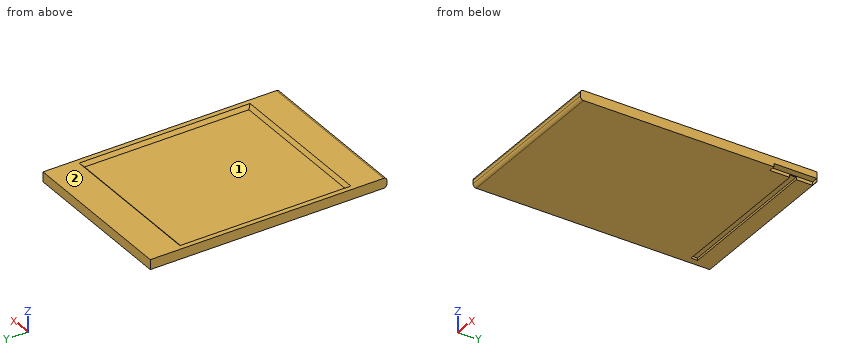
```python
from build123d import *

# Parameters (mm, degrees)
CROQUIS1_W              = 500
CROQUIS1_H              = 720
SALIENTE_EXTRUIR1_DEPTH = 30
CROQUIS2_W              = 450
CROQUIS2_H              = 500
CORTAR_EXTRUIR1_DEPTH   = 10
CHAFL_N1_SIZE           = 10
CHAFL_N2_SIZE           = 10
REDONDEO2_R             = 10
REDONDEO3_R             = 10
CROQUIS11_W             = 480
CROQUIS11_H             = 20
CORTAR_EXTRUIR5_DEPTH   = 7
CROQUIS12_W             = 10
CROQUIS12_H             = 130
CORTAR_EXTRUIR6_DEPTH   = 20


with BuildPart() as part:
    # Croquis1 → Saliente-Extruir1 (new body)
    with BuildSketch(Plane.XY):
        Rectangle(CROQUIS1_W, CROQUIS1_H)
    extrude(amount=SALIENTE_EXTRUIR1_DEPTH)

    # Croquis2 → Cortar-Extruir1 (cut)
    with BuildSketch(Plane.XY.offset(30)):
        Rectangle(CROQUIS2_W, CROQUIS2_H)
    extrude(amount=-CORTAR_EXTRUIR1_DEPTH, mode=Mode.SUBTRACT)

    # Chaflán1
    chafl_n1_edges = [part.edges().sort_by_distance(p)[0] for p in [
        (0, 250, 30),
    ]]
    chamfer(chafl_n1_edges, length=CHAFL_N1_SIZE - 0.0001)  # a hair under: the kernel refuses the full size

    # Chaflán2
    chafl_n2_edges = [part.edges().sort_by_distance(p)[0] for p in [
        (225, 4.99995, 30),
        (0, -250, 30),
        (-225, 4.99995, 30),
    ]]
    chamfer(chafl_n2_edges, length=CHAFL_N2_SIZE - 0.0001)  # a hair under: the kernel refuses the full size

    # Redondeo2
    redondeo2_edges = [part.edges().sort_by_distance(p)[0] for p in [
        (0, -360, 30),
    ]]
    fillet(redondeo2_edges, radius=REDONDEO2_R)

    # Redondeo3
    redondeo3_edges = [part.edges().sort_by_distance(p)[0] for p in [
        (0, -360, 0),
    ]]
    fillet(redondeo3_edges, radius=REDONDEO3_R)

    # Croquis11 → Cortar-Extruir5 (cut)
    with BuildSketch(Plane(origin=(0, 0, 0), x_dir=(-1, 0, 0), z_dir=(0, 0, -1))):
        with Locations((-10, 300)):
            Rectangle(CROQUIS11_W, CROQUIS11_H)
    extrude(amount=-CORTAR_EXTRUIR5_DEPTH, mode=Mode.SUBTRACT)

    # Croquis12 → Cortar-Extruir6 (cut)
    with BuildSketch(Plane(origin=(250, 0, 0), x_dir=(0, 0, -1), z_dir=(1, 0, 0))):
        with Locations((-5, 294.429232032)):
            Rectangle(CROQUIS12_W, CROQUIS12_H)
    extrude(amount=-CORTAR_EXTRUIR6_DEPTH, mode=Mode.SUBTRACT)


solid = part.part
```
Geometry: final body of the model. Coordinates: model frame, mm. Face numbers are marked on the shaded views. Coordinates: 2 decimals unless noted, no trailing zeros. Answer in a Markdown table with one row per item. Add a question column.
Q1. Mould query, pull axis Y, two halves, no side actions, for the marked faces 1 and 2. Classes: released by +Y, released by -Y, zero draft, split by the parting line, or undercut.
Q2. Contact query for flat-ended pins moving along their axis: P1, Ø8, axis at x = 238.5, z = 2.5, coming from the -Y side; P2, Ø7.5, axis at x = -49.5, z = 3, coming from the -Y side; P3, Ø8, axis at x = 85.5, y = 202, coming from the +Z side. Output: stop coordinate, or through.
Q3. Line query: L1, parallel to Z at x = 106, y = -189.5; L2, parallel to Y at x = -170, z = 6; L3, parallel to Y at x = 97.5, z = 26.5. Output: solid intervals per line, ascending.
Completed:
| question | item | result |
|---|---|---|
| 1 | face 1 | undercut |
| 1 | face 2 | zero draft |
| 2 | P1 | stops at y = -359.37 |
| 2 | P2 | stops at y = -359.46 |
| 2 | P3 | stops at z = 20 |
| 3 | L1 | z = 0 to 20 |
| 3 | L2 | y = -359.17 to 290, 310 to 360 |
| 3 | L3 | y = -357.6 to -256.5, 256.5 to 360 |
